Here's how the part is built. I have some questions about the finished solid (model axes, mm). A direction names the side the tool comes from. Give positions to 0.01 mm unless a question says otherwise; leave off trailing zeros. Loops run counter-clockwise (first coordinate to the right, second up) from the corner with the lowest first, then second, coordinate; pieces in that order, holes last. Notation, with made-up numbers: M 78,-31.75 L 116,-31.75 A26 cw 116,4.25 Z; hole C -27.75,65.5 d7. An arc over 180 degrees is marked long. Answer as CSV lines item,"result". Start each with the question number.
Item 1: For faces 1 (the flat face through (-1, -72, 0)), 2 (the flat face through (-1, -177.8, 50)), which set-ups out of +Z, -Z, +X, -X, +Y, -Y let a thin tool reach every point of the face, with its end or its side?
Item 2: I want a section at B-B on x = 0. List the corners of the cut face in (y, z) for me.
Item 3: Will these pins go through, and if not, where does the flat tip stop? P1, Ø8, axis at x = 22, z = 58.5, coming from the -Y side; P2, Ø1, axis at y = -42, z = 40, coming from the +X side; P3, Ø1.5, axis at x = -37.5, z = 71.5, coming from the +Y side.
Item 4: I want a section at A-A on y = 0. List the corners of the cut face in (x, z) for me, plus the area to 3 significant figures.
Item 5: If I drill on line 1 along Y through (x, z) = (1, 23); line 2 along X through (y, z) = (-11.5, 70); line 3 along X through (y, z) = (23.5, 13), over which ranges is the centre line in solid material (lowest first)? Write a range as from..to.
Item 6: If we mould it in two halves opening along X, with no side actions, what happens to faces 3 (the cylindrical face through (0.819, 50.793, 50.089)), 4 (the flat face through (53, -198.12, 50)), 5 (the flat face through (43.18, -188, 50))? For each: released by +X, released by -X, zero draft, split by the parting line, or undercut.
Item 7: I want a section at C-C on z = 48. List the corners of the cut face in (x, y) for me.
Item 8: I want a section at D-D on y = -78.5. List the corners of the cut face in (x, z) for me.
from build123d import *

# Parameters (mm, degrees)
SKETCH1_R           = 25.4
BOSS_EXTRUDE1_DEPTH = 101.6


with BuildPart() as part:
    # Sketch1 → Boss-Extrude1 (new body)
    with BuildSketch(Plane.XY):
        with BuildLine():
            Line((43.18, -177.8), (43.18, -198.12))
            Line((43.18, -198.12), (63.5, -198.12))
            Line((63.5, -198.12), (63.5, -122.435433935))
            ThreePointArc((63.5, -122.435433935), (36.049391603, -79.421078062), (41.89548787, -28.729916397))
            ThreePointArc((41.89548787, -28.729916397), (43.95358505, -24.826361045), (46.234198191, -21.048489675))
            ThreePointArc((46.234198191, -21.048489675), (-0.610127533, 50.796335935), (-45.715295245, -22.152918107))
            ThreePointArc((-45.715295245, -22.152918107), (-44.106525914, -24.87240035), (-42.611881246, -27.65623938))
            ThreePointArc((-42.611881246, -27.65623938), (-36.071200921, -78.724738597), (-63.5, -122.295750663))
            Line((-63.5, -122.295750663), (-63.5, -198.12))
            Line((-63.5, -198.12), (-43.18, -198.12))
            Line((-43.18, -198.12), (-43.18, -177.8))
            Line((-43.18, -177.8), (43.18, -177.8))
        make_face()
        Circle(SKETCH1_R, mode=Mode.SUBTRACT)
    extrude(amount=BOSS_EXTRUDE1_DEPTH)


solid = part.part
Result:
1,face 1,"-Z, +X, -X, +Y, -Y"
1,face 2,"+Z, -Z, -Y"
2,outline,"M -177.8,0 L -25.4,0 L -25.4,101.6 L -177.8,101.6 Z; M 25.4,0 L 50.8,0 L 50.8,101.6 L 25.4,101.6 Z"
3,P1,"y = -177.8"
3,P2,"x = 37"
3,P3,"y = 35.07"
4,outline,"M -50.8,0 L -25.4,0 L -25.4,101.6 L -50.8,101.6 Z; M 25.4,0 L 50.8,0 L 50.8,101.6 L 25.4,101.6 Z"
4,area,"5,160 mm^2"
5,line 1,"-177.8..-25.38, 25.38..50.79"
5,line 2,"-49.48..-22.65, 22.65..49.48"
5,line 3,"-45.04..-9.64, 9.64..45.04"
6,face 3,"split by the parting line"
6,face 4,"zero draft"
6,face 5,"undercut"
7,outline,"M -63.5,-198.12 L -43.18,-198.12 L -43.18,-177.8 L 43.18,-177.8 L 43.18,-198.12 L 63.5,-198.12 L 63.5,-122.44 A76.2 cw 46.23,-21.05 A50.8 ccw long -45.72,-22.15 A76.2 cw -63.5,-122.3 Z; hole C 0,0 d50.8"
8,outline,"M -36.02,0 L 35.84,0 L 35.84,101.6 L -36.02,101.6 Z"
